from build123d import *

# Parameters (mm, degrees)
FILLET1_R = 5


with BuildPart() as part:
    # Sketch1 → Revolve1 (revolve)
    with BuildSketch(Plane(origin=(0, 0, 0), x_dir=(1, 0, 0), z_dir=(0, 1, 0))):
        Polygon((1040, 0), (-1040, 0), (-1040, 50), (-950, 50), (-950, 150), (950, 150), (950, 50), (1040, 50), align=None)
    revolve(axis=Axis((1040, 0, 0), (-1, 0, 0)))

    # Fillet1
    fillet1_edges = [part.edges().sort_by_distance(p)[0] for p in [
        (-950, 0, 50),
        (950, 0, 50),
    ]]
    fillet(fillet1_edges, radius=FILLET1_R)


solid = part.part
Input: part model. Units: mm. Frame: model coordinates. A direction names the side the tool comes from. Coordinates: 2 decimals unless noted, no trailing zeros. Loops run counter-clockwise (first coordinate to the right, second up) from the corner with the lowest first, then second, coordinate; pieces in that order, holes last. Notation, with made-up numbers: (68, 81.5) -> (77, 81.5) arc R18 cw to (77, 107.5) -> close; hole circle Ø1 at (24.5, 81). An arc over 180 degrees is marked (long way). One line per item, written item: value.
(1) Cut plane A-A (z = 0). Output: boundary loops of the cut face in (x, y), then the cut area to 3 significant figures.
Answer below:
outline: (-1040, -50) -> (-955, -50) arc R5 cw to (-950, -55) -> (-950, -150) -> (950, -150) -> (950, -55) arc R5 cw to (955, -50) -> (1040, -50) -> (1040, 50) -> (955, 50) arc R5 cw to (950, 55) -> (950, 150) -> (-950, 150) -> (-950, 55) arc R5 cw to (-955, 50) -> (-1040, 50) -> close
area: 588,000 mm2
(2) Cut plane C-C (x = 180). Output: boundary loops of the cut face in (y, z).
Answer below:
outline: circle Ø300 at (0, 0)
(3) Set-up query: faces 1 (the face through (-996.9, -15.02, -47.69)), 2 (the face through (998.1, -15.02, -47.69)), 3 (the face through (1040, -1, 1)). Return all of +Z, -Z, +X, -X, +Y, -Y with unobstructed straight access to the full face (end or side cutting, diameter ignored); none if empty.
Answer below:
face 1: -X
face 2: +X
face 3: +Z, -Z, +X, +Y, -Y
(4) Ray query, line 1 along X through (y, z) = (-81, -36.5); line 2 along Y through (x, z) = (-394, 3); line 3 along Z through (x, y) = (-555.5, -9). Return the intervals inside material, ascending.
Answer below:
line 1: x = -950 to 950
line 2: y = -149.97 to 149.97
line 3: z = -149.73 to 149.73
(5) Pin query (flat end, axial travel): pin 1 Ø1.5 at (x, z) = (405.5, -117.5) entering from +Y; pin 2 Ø5 at (y, z) = (-58.5, 57.5) entering from -X; pin 3 Ø1 at (x, y) = (-84.5, 75) entering from +Z. Return the tip coordinate at first contact, or that it passes through.
Answer below:
pin 1: stops at y = 94.18
pin 2: stops at x = -950
pin 3: stops at z = 130.19
(6) Cut plane D-D (y = 84). Output: boundary loops of the cut face in (x, z), then the cut area to 3 significant figures.
Answer below:
outline: (-950, -124.27) -> (950, -124.27) -> (950, 124.27) -> (-950, 124.27) -> close
area: 472,000 mm2
